Can you work these out from the model? Positions are in its coordinate system, mm. A direction names the side the tool comes from. Give positions to 0.01 mm unless a question says otherwise; leave off trailing zeros. Loops run counter-clockwise (first coordinate to the right, second up) from the corner with the lowest first, then second, coordinate; pieces in that order, holes last. Notation, with made-up numbers: (43.5, 44.5) - (85.5, 44.5) arc R30 cw to (85.5, 68.5) - close; hole circle Ø9 at (15.25, 47.5). An arc over 180 degrees is marked (long way). Answer in a Markdown table with one row per item.
from build123d import *

# Parameters (mm, degrees)
SKETCH2_R           = 20
BOSS_EXTRUDE1_DEPTH = 4.3


with BuildPart() as part:
    # Sketch2 → Boss-Extrude1 (new body)
    with BuildSketch(Plane.XY):
        Polygon((0, 0), (6.693, 0), (6.693, 4.7), (21.693, 4.7), (21.693, 0), (33.136, 0), (33.136, 4.7), (48.136, 4.7), (48.136, 0), (59.579, 0), (59.579, 4.7), (74.579, 4.7), (74.579, 0), (86.022, 0), (86.022, 4.7), (101.022, 4.7), (101.022, 0), (112.465, 0), (112.465, 4.7), (127.465, 4.7), (127.465, 0), (138.908, 0), (138.908, 4.7), (153.908, 4.7), (153.908, 0), (160.6, 0), (160.6, 13.575), (165.3, 13.575), (165.3, 28.875), (160.6, 28.875), (160.6, 42.35), (165.3, 42.35), (165.3, 57.65), (160.6, 57.65), (160.6, 71.125), (165.3, 71.125), (165.3, 86.425), (160.6, 86.425), (160.6, 100), (154.058, 100), (154.058, 104.7), (138.758, 104.7), (138.758, 100), (127.615, 100), (127.615, 104.7), (112.315, 104.7), (112.315, 100), (101.172, 100), (101.172, 104.7), (85.872, 104.7), (85.872, 100), (74.729, 100), (74.729, 104.7), (59.429, 104.7), (59.429, 100), (48.286, 100), (48.286, 104.7), (32.986, 104.7), (32.986, 100), (21.843, 100), (21.843, 104.7), (6.543, 104.7), (6.543, 100), (0, 100), (0, 86.425), (-4.7, 86.425), (-4.7, 71.125), (0, 71.125), (0, 57.65), (-4.7, 57.65), (-4.7, 42.35), (0, 42.35), (0, 28.875), (-4.7, 28.875), (-4.7, 13.575), (0, 13.575), align=None)
        with Locations(Location((55, 70, 0), (0, 0, 180))):
            Circle(SKETCH2_R, mode=Mode.SUBTRACT)
    extrude(amount=BOSS_EXTRUDE1_DEPTH)


solid = part.part
Q1. For pin 1 (1.3 mm diameter, centred on x = 2, z = 3, fed in from +Y); pin 2 (1.3 mm diameter, centred on x = -1.5, z = 1.5, fed in from +Y) (3 decimals); pin 3 (2 mm diameter, centred on x = 163, z = 3, fed in from -Y) (3 decimals), each with a flat end and sliding along its axis, tell me the tip position at first contact or that it passes through.
Checked values:
| item | result |
|---|---|
| pin 1 | stops at y = 100 |
| pin 2 | stops at y = 86.425 |
| pin 3 | stops at y = 13.575 |
Q2. On a 3-axis mill with a long thin cutter (end or side, diameter ignored), from which of +Z, -Z, +X, -X, +Y, -Y can I reach the whole of each face in a straight line? I mean faces 1 (the face through (59.429, 102, 2)), 2 (the face through (-4.7, 79, 2)), 3 (the face through (74.579, 2, 2)), 4 (the face through (-2, 28.875, 2)), 5 (the face through (3, 100, 2)). Say none if no direction works.
Checked values:
| item | result |
|---|---|
| face 1 | +Z, -Z, +Y |
| face 2 | +Z, -Z, -X, +Y, -Y |
| face 3 | +Z, -Z, -Y |
| face 4 | +Z, -Z, -X |
| face 5 | +Z, -Z, -X, +Y |
Q3. Imagine slicing it at B-B, the plane y = 79. Write out the boundary of the cut face in (x, z), and give its area (3 significant figures).
Checked values:
| item | result |
|---|---|
| outline | (-4.7, 0) - (37.14, 0) - (37.14, 4.3) - (-4.7, 4.3) - close; (72.86, 0) - (165.3, 0) - (165.3, 4.3) - (72.86, 4.3) - close |
| area | 577 mm² |
Q4. Imagine slicing it at A-A, the plane x = 55. Write out the boundary of the cut face in (y, z), and give its area (3 significant figures).
Checked values:
| item | result |
|---|---|
| outline | (0, 0) - (50, 0) - (50, 4.3) - (0, 4.3) - close; (90, 0) - (100, 0) - (100, 4.3) - (90, 4.3) - close |
| area | 258 mm² |
Q5. Imagine slicing it at C-C, the plane x = 151. Write out the boundary of the cut face in (y, z).
Checked values:
| item | result |
|---|---|
| outline | (4.7, 0) - (104.7, 0) - (104.7, 4.3) - (4.7, 4.3) - close |
Q6. If I drill on line 1 (X direction, y = 70, z = 2.5); line 2 (Y direction, x = 55, z = 1.1); line 3 (X direction, y = 30, z = 3.9), over which ranges is the centre line in solid material (lowest first)? Write a range as [from, to].
Checked values:
| item | result |
|---|---|
| line 1 | x = [0, 35], [75, 160.6] |
| line 2 | y = [0, 50], [90, 100] |
| line 3 | x = [0, 160.6] |
Q7. If we mould it in two halves opening along Y, with no side actions, what happens to faces 6 (the face through (112.315, 102, 2)), 7 (the face through (94, 104.7, 2)), 8 (the face through (163, 42.35, 2))? For each: released by +Y, released by -Y, zero draft, split by the parting line, or undercut.
Checked values:
| item | result |
|---|---|
| face 6 | zero draft |
| face 7 | released by +Y |
| face 8 | undercut |
Q8. Imagine slicing it at D-D, the plane y = 32. Write out the boundary of the cut face in (x, z).
Checked values:
| item | result |
|---|---|
| outline | (0, 0) - (160.6, 0) - (160.6, 4.3) - (0, 4.3) - close |
